from build123d import *

# Parameters (mm, degrees)
CUT_EXTRUDE_1_DEPTH      = 23.869193331
CUT_EXTRUDE_1_DEPTH_BACK = 23.869193331
SKETCH_2_R               = 1


with BuildPart() as part:
    # Эскиз1 → Повернуть1 (revolve)
    with BuildSketch(Plane.XY, mode=Mode.PRIVATE) as revolve_1_sk:
        with BuildLine():
            Line((0, 3), (0, 4.5))
            Line((0, 4.5), (6, 4.5))
            Line((6, 4.5), (6, 9))
            Line((6, 9), (9.9, 9))
            ThreePointArc((9.9, 9), (9.970710678, 8.970710678), (10, 8.9))
            Line((10, 8.9), (10, 7.6))
            ThreePointArc((10, 7.6), (10.146446609, 7.246446609), (10.5, 7.1))
            Line((10.5, 7.1), (13, 7.1))
            ThreePointArc((13, 7.1), (13.353553391, 7.246446609), (13.5, 7.6))
            Line((13.5, 7.6), (13.5, 8.9))
            ThreePointArc((13.5, 8.9), (13.529289322, 8.970710678), (13.6, 9))
            Line((13.6, 9), (19, 9))
            Line((19, 9), (19, 8.5))
            Line((19, 8.5), (17.526279442, 3))
            Line((17.526279442, 3), (0, 3))
        make_face()
    revolve(revolve_1_sk.sketch.rotate(Axis((0, 0, 0), (1, 0, 0)), 90), axis=Axis((0, 0, 0), (1, 0, 0)))

    # Эскиз2 → Вырез-Вытянуть1 (cut, two sides: drawn at the far end of the back side and taken through both)
    with BuildSketch(Plane(origin=(0, 0, 0), x_dir=(1, 0, 0), z_dir=(0, 1, 0)).offset(-CUT_EXTRUDE_1_DEPTH_BACK)):
        with Locations(Location((3, 0, 0), (0, 0, 270))):
            Circle(SKETCH_2_R)
    extrude(amount=CUT_EXTRUDE_1_DEPTH + CUT_EXTRUDE_1_DEPTH_BACK, mode=Mode.SUBTRACT)


solid = part.part
The model under review builds one solid part; all positions refer to its coordinate system, in mm. A direction names the side the tool comes from. Give positions to 0.01 mm unless a question says otherwise; leave off trailing zeros. Write each loop counter-clockwise with the first axis right and the second up, starting at its lowest first coordinate (ties: lowest second). Pieces come first, ordered by that corner, then holes.
1. Tool access review of faces 4 (the flat face through (10, -4, 7)), 5 (the cylindrical face through (3, -4, -1)), 6 (the flat face through (6, 4, -4)): name each direction out of +Z, -Z, +X, -X, +Y, -Y from which nothing blocks a thin tool from reaching the whole face with its end or side.
2. Draft analysis for pull direction X (two halves, no side actions). For faces 1 (the conical face through (17.6, 3.2, -0.7)), 2 (the cylindrical face through (16.338, -6.083, -6.633)), 3 (the cylindrical face through (11.77, -7.04, -0.92)), state which applies: +X half, -X half, draft (parallel to the pull), parting line (faces both ways), or undercut.
3. Add section C-C, the plane z = 0. Count the separate pieces of the cut face and the enclosed holes in it, plus the area to 3 significant figures.
4. Wall thickness on L1, parallel to Y at x = 13.75, z = 0; L2, parallel to Y at x = 10.75, z = 0; L3, parallel to X at y = -8, z = 0.25: over which ranges is each line inside the solid? List them lowest first.
5. For P1, Ø3, axis at x = 3, z = 0, coming from the +Y side; P2, Ø5.5, axis at y = 2.5, z = 1, coming from the +X side; P3, Ø7, axis at y = 0, z = 0, coming from the +X side, all flat-tipped, find the tip position at first contact; note any pin that passes through.
6. Add section D-D, the plane x = 6.5. Write out the cut boundary in (y, z).
7. Add section B-B, the plane x = 3. Write out the cut boundary in (y, z), plus the area to 3 significant figures.
Worked answers:
1. face 4: none
1. face 5: +Y, -Y
1. face 6: -X
2. face 1: +X half
2. face 2: draft
2. face 3: undercut
3. separate pieces: 4
3. enclosed holes: 0
3. area: 147 mm2
4. L1: y = -9 to -3, 3 to 9
4. L2: y = -7.1 to -3, 3 to 7.1
4. L3: x = 6 to 10, 13.5 to 18.87
5. P1: stops at y = 4.5
5. P2: stops at x = 18.18
5. P3: stops at x = 17.66
6. outline: circle Ø18 at (0, 0); hole circle Ø6 at (0, 0)
7. outline: (-4.39, -1) arc R4.5 ccw to (4.39, -1) - (2.83, -1) arc R3 cw to (-2.83, -1) - close; (-4.39, 1) - (-2.83, 1) arc R3 cw to (2.83, 1) - (4.39, 1) arc R4.5 ccw to start
7. area: 29.3 mm2
